Geometry check sheet. Reference: the model listing, model coordinates, mm. Face numbers are marked on the shaded views. A direction names the side the tool comes from. Round coordinates to 2 decimals unless told otherwise and drop trailing zeros. Write each loop counter-clockwise with the first axis right and the second up, starting at its lowest first coordinate (ties: lowest second). Pieces come first, ordered by that corner, then holes. Notation, with made-up numbers: M 82.5,70.5 L 121.5,70.5 A22 ccw 121.5,97.5 Z; hole C 18.5,59.25 d11. An arc over 180 degrees is marked long. One line per item, written item: value. Start each with the question number.
1. Section check B-B (z = 65). Record the boundary of the cut face in (x, y).
2. Depth check by flat-ended pin: P1, Ø17.5, axis at y = 27, z = 59, coming from the +X side; P2, Ø11.5, axis at x = -3, y = 43.5, coming from the +Z side; P3, Ø12, axis at y = 46.5, z = 62, coming from the -X side. Enter the tip coordinate at first touch or a pass-through.
3. Section check A-A (y = 26). Record the boundary of the cut face in (x, z).
4. Section check C-C (x = -1.5). Record the boundary of the cut face in (y, z), and give its area (3 significant figures).
5. Section check D-D (y = 4.5). Record the boundary of the cut face in (x, z), and give its area (3 significant figures).
6. Scan lines: probe 1 along Y at (x, z) = (-6, 54.5); probe 2 along Y at (x, z) = (10, 97); probe 3 along Z at (x, y) = (-23.5, 4.5). Record each from-to range of solid material in increasing order. Write a range as [from, to].
7. Access from +Z, -Z, +X, -X, +Y, -Y to the whole of each face (thin tool, end or side, straight path). Record for the marked faces 1, 2, 3 and 4.
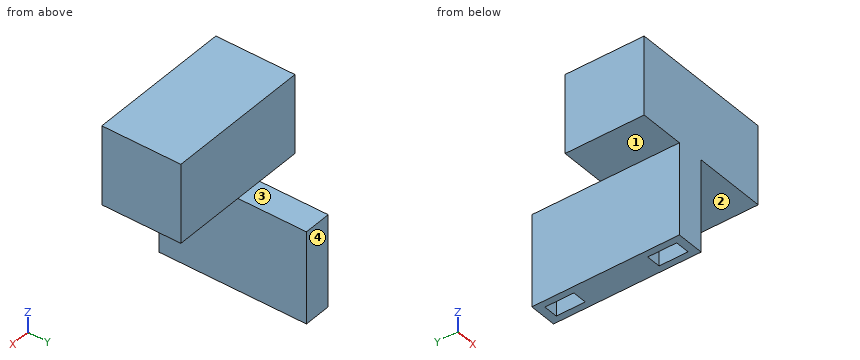
from build123d import *

# Parameters (mm, degrees)
SKETCH1_W           = 55
SKETCH1_H           = 30
BOSS_EXTRUDE1_DEPTH = 30
SKETCH2_W           = 10.5
SKETCH2_H           = 56
BOSS_EXTRUDE2_DEPTH = 35
SKETCH3_W           = 5.5
SKETCH3_H           = 11
CUT_EXTRUDE1_DEPTH  = 22


with BuildPart() as part:
    # Sketch1 → Boss-Extrude1 (new body)
    with BuildSketch(Plane(origin=(0, 0, 0), x_dir=(1, 0, 0), z_dir=(0, 1, 0))):
        Rectangle(SKETCH1_W, SKETCH1_H)
    extrude(amount=BOSS_EXTRUDE1_DEPTH)

    # Sketch2 → Boss-Extrude2 (add)
    with BuildSketch(Plane.XY.offset(15)):
        with Locations((-5.25, 28)):
            Rectangle(SKETCH2_W, SKETCH2_H)
    extrude(amount=BOSS_EXTRUDE2_DEPTH)

    # Sketch3 → Cut-Extrude1 (cut)
    with BuildSketch(Plane.XY.offset(50)):
        with Locations((-5.25, 8.5)):
            Rectangle(SKETCH3_W, SKETCH3_H)
        with Locations((-5.25, 47.5)):
            Rectangle(SKETCH3_W, SKETCH3_H)
    extrude(amount=-CUT_EXTRUDE1_DEPTH, mode=Mode.SUBTRACT)


with BuildPart() as body_2:
    # Mirror1: mirrored copy
    add(part.part.mirror(Plane.XY.offset(50)))


solid = body_2.part
Result sheet:
1. outline: M -10.5,0 L 0,0 L 0,56 L -10.5,56 Z; hole M -8,3 L -2.5,3 L -2.5,14 L -8,14 Z; hole M -8,42 L -2.5,42 L -2.5,53 L -8,53 Z
2. P1: stops at x = 0
2. P2: stops at z = 85
2. P3: stops at x = -10.5
3. outline: M -27.5,85 L -10.5,85 L -10.5,50 L 0,50 L 0,85 L 27.5,85 L 27.5,115 L -27.5,115 Z
4. outline: M 0,50 L 56,50 L 56,85 L 30,85 L 30,115 L 0,115 Z
4. area: 2,860 mm2
5. outline: M -27.5,85 L -10.5,85 L -10.5,50 L -8,50 L -8,72 L -2.5,72 L -2.5,50 L 0,50 L 0,85 L 27.5,85 L 27.5,115 L -27.5,115 Z
5. area: 1,900 mm2
6. probe 1: y = [0, 3], [14, 42], [53, 56]
6. probe 2: y = [0, 30]
6. probe 3: z = [85, 115]
7. face 1: -Z, -X, +Y, -Y
7. face 2: -Z, +X, +Y, -Y
7. face 3: +Z, +X, -X, +Y
7. face 4: +Z, -Z, +X, -X, +Y
